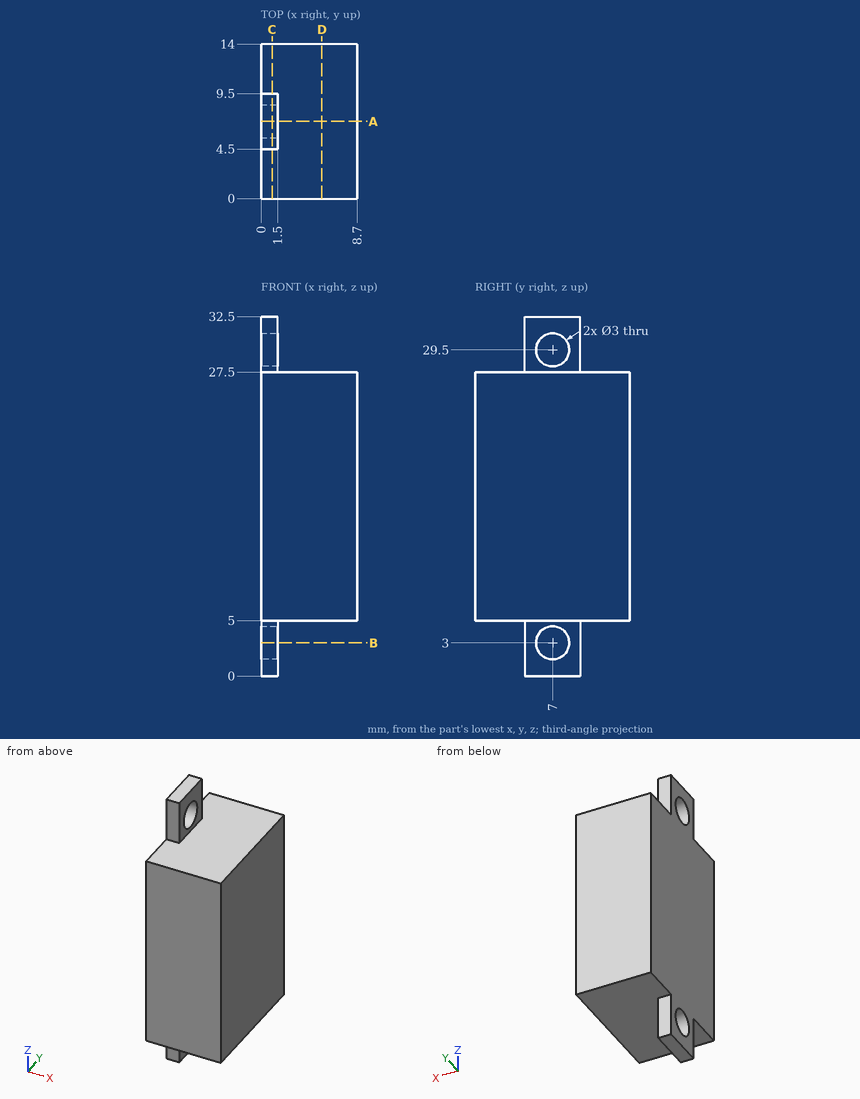
Input: dimensioned drawing with shaded views. Units: mm. Origin: part minimum x, y, z. Give positions to 0.01 mm unless a question says otherwise; leave off trailing zeros. Write each loop counter-clockwise with the first axis right and the second up, starting at its lowest first coordinate (ties: lowest second). Pieces come first, ordered by that corner, then holes. Notation, with made-up numbers: (60.5, 15) - (106.5, 15) arc R18 ccw to (106.5, 23) - close; hole circle Ø8 at (20, 57.25). An arc over 180 degrees is marked (long way). Write item = value, one per line. Start each with the question number.
1) Cut plane C-C (x = 1). Return loops of the section in (y, z), and give its area (3 significant figures).
2) Pin query (flat end, axial travel): pin 1 (2.5 mm diameter, centred on x = 2.5, y = 9, fed in from +Z); pin 2 (4 mm diameter, centred on y = 7, z = 30.5, fed in from +X); pin 3 (1.2 mm diameter, centred on x = 0.5, z = 29, fed in from -Y); pin 4 (1.8 mm diameter, centred on y = 7, z = 29.5, fed in from +X). Return the tip coordinate at first contact, or that it passes through.
3) Cut plane A-A (y = 7). Return loops of the section in (x, z), and give its area (3 significant figures).
4) Cut plane B-B (z = 3). Return loops of the section in (x, y).
5) Cut plane D-D (x = 5.5). Return loops of the section in (y, z).
6) Material intervals for L1, parallel to Z at x = 0.4, y = 7; L2, parallel to Y at x = 0.9, z = 3; L3, parallel to Z at x = 2.75, y = 5.5, sorted ascending. Write a range as [from, to].
Answers follow:
q1.outline = (0, 5) - (4.5, 5) - (4.5, 0) - (9.5, 0) - (9.5, 5) - (14, 5) - (14, 27.5) - (9.5, 27.5) - (9.5, 32.5) - (4.5, 32.5) - (4.5, 27.5) - (0, 27.5) - close; hole circle Ø3 at (7, 3); hole circle Ø3 at (7, 29.5)
q1.area = 351 mm^2
q2.pin_1 = 32.5
q2.pin_2 = 1.5
q2.pin_3 = 4.5
q2.pin_4 = through
q3.outline = (0, 0) - (1.5, 0) - (1.5, 1.5) - (0, 1.5) - close; (0, 4.5) - (1.5, 4.5) - (1.5, 5) - (8.7, 5) - (8.7, 27.5) - (1.5, 27.5) - (1.5, 28) - (0, 28) - close; (0, 31) - (1.5, 31) - (1.5, 32.5) - (0, 32.5) - close
q3.area = 202 mm^2
q4.outline = (0, 4.5) - (1.5, 4.5) - (1.5, 5.5) - (0, 5.5) - close; (0, 8.5) - (1.5, 8.5) - (1.5, 9.5) - (0, 9.5) - close
q5.outline = (0, 5) - (14, 5) - (14, 27.5) - (0, 27.5) - close
q6.L1 = [0, 1.5], [4.5, 28], [31, 32.5]
q6.L2 = [4.5, 5.5], [8.5, 9.5]
q6.L3 = [5, 27.5]
